Part model, mm, in its own coordinate system. A direction names the side the tool comes from. Coordinates: 2 decimals unless noted, no trailing zeros. Order: outer loops, then holes, each group sorted by start corner. A loop starts at its lowest first (then second) coordinate and runs counter-clockwise, first axis right, second up.
1) Tool access for faces 1 (the flat face through (-19, -60.715, 4)), 2 (the flat face through (22.37, -21, 4)), 3 (the cylindrical face through (27.41, -41.78, 4.02)): list every direction of +Z, -Z, +X, -X, +Y, -Y with a clear straight run to the whole face (end or side of a thin tool).
2) Cut at C-C (y = 23.5). List the corners of the cut face in (x, z).
3) Wall check: L1, parallel to X at y = -8.5, z = 7; L2, parallel to Y at x = 24, z = 1.25; L3, parallel to X at y = 24, z = 3.25. Give the ranges that are in metal, low to high.
4) Cut at A-A (y = -32.5). List the corners of the cut face in (x, z), and give its area (3 significant figures).
5) Cut at B-B (z = 3). List the corners of the cut face in (x, y) (3 decimals).
6) Mould opens along X. For faces 4 (the flat face through (38.245, -11, 4)), 5 (the flat face through (30, -60.715, 4)), 6 (the cylindrical face through (-4.896, -41.554, 4.024)) say: +X half, -X half, draft (parallel to the pull), parting line (faces both ways), or undercut.
7) Pin check, flat tip, straight feed: pin 1 Ø11.5 at (x, y) = (-22.57, 0) entering from -Z. Stop position of the tip, or through.
```python
from build123d import *

# Parameters (mm, degrees)
F0_W     = 12.7
F0_H     = 19.05
F1_DEPTH = 7.9375
F2_D     = 10.0838
F3_D     = 13.49248


# Not quite as in the source:
# - a feature names something its author has since deleted; it is built from what else it names


with BuildPart() as f1:
    # F0 (on Top) → F1 (new body)
    with BuildSketch(Plane.XY):
        Polygon((25.5451762405, 40.8851695299), (-25.2548237595, 40.8851695299), (-25.2548237595, 21.8351695299), (-37.9548237595, 21.8351695299), (-37.9548237595, -60.7148304701), (0.1451762405, -60.7148304701), (0.1451762405, -41.6648304701), (0.1451762405, -0.3898304701), (22.3701762405, -0.3898304701), (22.3701762405, -41.6648304701), (22.3701762405, -60.7148304701), (38.2451762405, -60.7148304701), (38.2451762405, 21.8351695299), (25.5451762405, 21.8351695299), align=None)
        with Locations((-31.6048237595, 31.3601695299)):
            Rectangle(F0_W, F0_H)
        with Locations((31.8951762405, 31.3601695299)):
            Rectangle(F0_W, F0_H)
    extrude(amount=F1_DEPTH)

    # F2 (through all)
    with Locations(Plane(origin=(0, 0, 0), x_dir=(1, 0, 0), z_dir=(0, 0, -1))):
        with Locations((0.1451762405, 0.3898304701), (0.1451762405, 41.6648304701), (-22.5665104002, 0), (-22.5665104002, 41.275), (22.3701762405, 41.6648304701), (22.3701762405, 0.3898304701)):
            Hole(F2_D / 2)

    # F3 (through all)
    with Locations(Plane(origin=(0, 0, 0), x_dir=(1, 0, 0), z_dir=(0, 0, -1))):
        with Locations((-25.2548237595, -21.8351695299), (25.5451762405, -21.8351695299)):
            Hole(F3_D / 2)


solid = f1.part
```
Geometry check:
1. face 1: +Z, -Z, +X, -X, -Y
1. face 2: +Z, -Z, -Y
1. face 3: +Z, -Z
2. outline: (-37.95, 0) - (-31.79, 0) - (-31.79, 7.94) - (-37.95, 7.94) - close; (-18.72, 0) - (19.01, 0) - (19.01, 7.94) - (-18.72, 7.94) - close; (32.08, 0) - (38.25, 0) - (38.25, 7.94) - (32.08, 7.94) - close
3. L1: x = -37.95 to 0.15, 22.37 to 38.25
3. L2: y = -60.71 to -46.44, -36.89 to -5.16, 4.38 to 15.27, 28.4 to 40.89
3. L3: x = -37.95 to -31.64, -18.87 to 19.16, 31.93 to 38.25
4. outline: (-37.95, 0) - (0.15, 0) - (0.15, 7.94) - (-37.95, 7.94) - close; (22.37, 0) - (38.25, 0) - (38.25, 7.94) - (22.37, 7.94) - close
4. area: 428 mm2
5. outline: (-37.955, -60.715) - (0.145, -60.715) - (0.145, -46.707) arc R5.042 cw to (0.145, -36.623) - (0.145, -5.432) arc R5.042 cw (long way) to (5.187, -0.39) - (17.328, -0.39) arc R5.042 cw (long way) to (22.37, -5.432) - (22.37, -36.623) arc R5.042 cw to (22.37, -46.707) - (22.37, -60.715) - (38.245, -60.715) - (38.245, 40.885) - (-37.955, 40.885) - close; hole circle Ø13.492 at (-25.255, 21.835); hole circle Ø10.084 at (-22.567, -41.275); hole circle Ø10.084 at (-22.567, 0); hole circle Ø13.492 at (25.545, 21.835)
6. face 4: +X half
6. face 5: draft
6. face 6: undercut
7. pin 1: stops at z = 0
